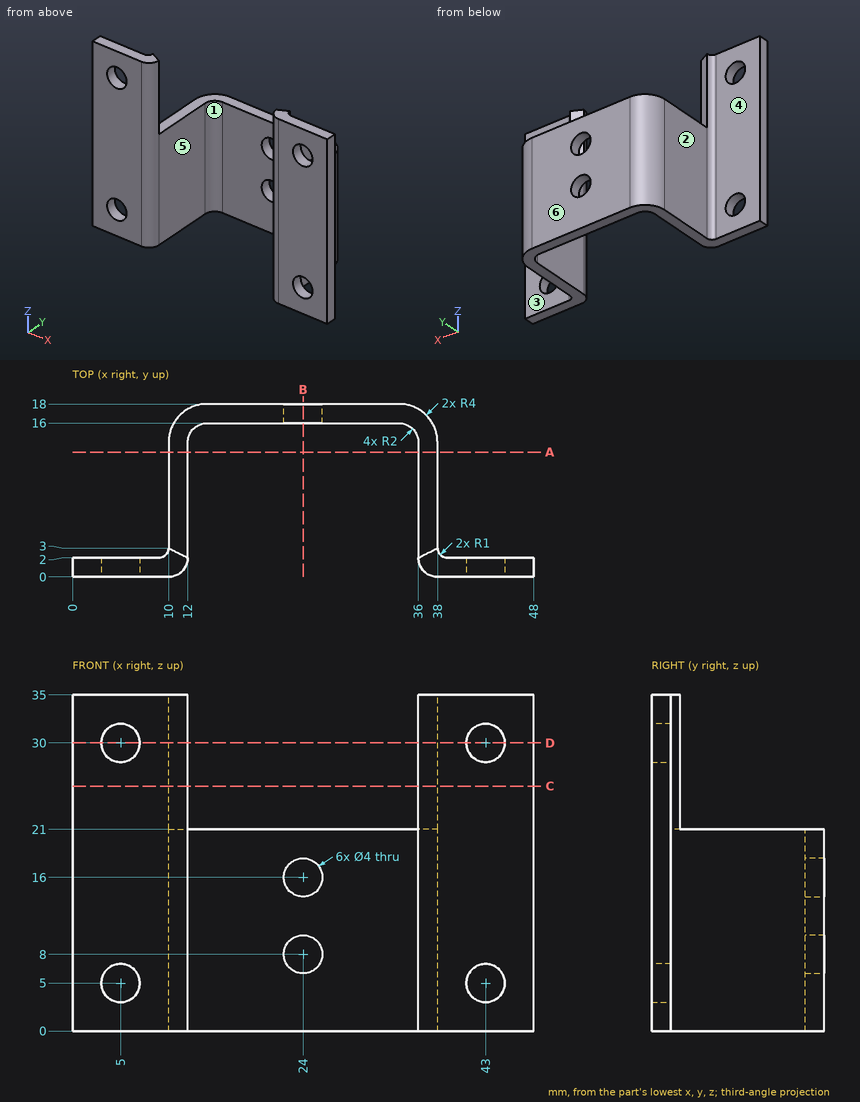
Geometry: see drawing. Coordinates: mm, zero at the bounding-box minimum. A direction names the side the tool comes from. Coordinates: 2 decimals unless noted, no trailing zeros. Loops run counter-clockwise (first coordinate to the right, second up) from the corner with the lowest first, then second, coordinate; pieces in that order, holes last.
Q1. Contact query for flat-ended pins moving along their axis: pin 1 (3 mm diameter, centred on x = 40.5, z = 10.5, fed in from +Y); pin 2 (10 mm diameter, centred on x = 21, z = 13.5, fed in from -Y); pin 3 (8 mm diameter, centred on y = 13, z = 21, fed in from +X). Output: stop coordinate, or through.
Q2. Cut plane A-A (y = 13). Output: boundary loops of the cut face in (x, z), then the cut area to 3 significant figures.
Q3. Set-up query: the marked faces 4, 5 and 6. Return all of +Z, -Z, +X, -X, +Y, -Y with unobstructed straight access to the full face (end or side cutting, diameter ignored); none if empty.
Q4. Cut plane C-C (z = 25.5). Output: boundary loops of the cut face in (x, y), then the cut area to 3 significant figures.
Q5. Cut plane B-B (x = 24). Output: boundary loops of the cut face in (y, z), then the cut area to 3 significant figures.
Q6. Draft query along X for the marked faces 1, 2 and 3. Return one class per face: +X half, -X half, draft (parallel to the pull), parting line (faces both ways), or undercut.
Q7. Cut plane D-D (z = 30). Output: boundary loops of the cut face in (x, y), then the cut area to 3 significant figures.
Q8. Material intervals for line 1 (Z direction, x = 43, y = 1.25); line 2 (X direction, y = 8, z = 7); line 3 (X direction, y = 1.15, z = 30), sorted ascending.
Working result:
1. pin 1: stops at y = 2
1. pin 2: stops at y = 16
1. pin 3: stops at x = 38
2. outline: (10, 0) - (12, 0) - (12, 21) - (10, 21) - close; (36, 0) - (38, 0) - (38, 21) - (36, 21) - close
2. area: 84.0 mm2
3. face 4: +Z, -Z, -X, +Y
3. face 5: +Z, -Z, -Y
3. face 6: +Z, -Z, +X, -X, +Y
4. outline: (0, 0) - (10, 0) arc R2 ccw to (12, 2) - (10, 3) arc R1 cw to (9, 2) - (0, 2) - close; (36, 2) arc R2 ccw to (38, 0) - (48, 0) - (48, 2) - (39, 2) arc R1 cw to (38, 3) - close
4. area: 48.7 mm2
5. outline: (16, 0) - (18, 0) - (18, 6) - (16, 6) - close; (16, 10) - (18, 10) - (18, 14) - (16, 14) - close; (16, 18) - (18, 18) - (18, 21) - (16, 21) - close
5. area: 26.0 mm2
6. face 1: undercut
6. face 2: -X half
6. face 3: draft
7. outline: (0, 0) - (3, 0) - (3, 2) - (0, 2) - close; (7, 0) - (10, 0) arc R2 ccw to (12, 2) - (10, 3) arc R1 cw to (9, 2) - (7, 2) - close; (36, 2) arc R2 ccw to (38, 0) - (41, 0) - (41, 2) - (39, 2) arc R1 cw to (38, 3) - close; (45, 0) - (48, 0) - (48, 2) - (45, 2) - close
7. area: 32.7 mm2
8. line 1: z = 0 to 3, 7 to 28, 32 to 35
8. line 2: x = 10 to 12, 36 to 38
8. line 3: x = 0 to 3, 7 to 11.81, 36.19 to 41, 45 to 48
